Here's how the part is built. I have some questions about the finished solid (model axes, mm). Face numbers are marked on the shaded views. A direction names the side the tool comes from. Round coordinates to 2 decimals unless told otherwise and drop trailing zeros. Order: outer loops, then holes, each group sorted by start corner. A loop starts at its lowest first (then second) coordinate and runs counter-clockwise, first axis right, second up. Notation, with made-up numbers: (85.25, -3) -> (132.25, -3) arc R15 cw to (132.25, 10) -> close; hole circle Ø4 at (7.25, 30). An arc over 180 degrees is marked (long way). One line per item, written item: value.
```python
from build123d import *

# Parameters (mm, degrees)
BOSS_EXTRUDE1_DEPTH = 12.7
SKETCH4_W           = 86.8
SKETCH4_H           = 86.8
SKETCH4_R           = 25.4
BOSS_EXTRUDE3_DEPTH = 340
SKETCH6_W           = 86.8
SKETCH6_H           = 62
CUT_EXTRUDE3_DEPTH  = 12
SKETCH7_W           = 62
SKETCH7_H           = 74.8
CUT_EXTRUDE4_DEPTH  = 12
SKETCH8_W           = 62
SKETCH8_H           = 74.8
CUT_EXTRUDE5_DEPTH  = 12
FILLET2_R           = 35


with BuildPart() as part:
    # Sketch1 → Boss-Extrude1 (new body)
    with BuildSketch(Plane(origin=(0, 0, 0), x_dir=(1, 0, 0), z_dir=(0, 1, 0))):
        Polygon((-367.549574024, 171.211944752), (132.450425976, 171.211944752), (132.450425976, -168.788055248), (-367.549574024, -168.788055248), (-367.549574024, -82.788055248), (7.450425976, -82.788055248), (7.450425976, 85.211944752), (-367.549574024, 85.211944752), align=None)
    extrude(amount=BOSS_EXTRUDE1_DEPTH)

    # Sketch4 → Boss-Extrude3 (add)
    with BuildSketch(Plane.XY.offset(168.788055248)):
        with Locations((50.850425976, 56.1)):
            Rectangle(SKETCH4_W, SKETCH4_H)
        with Locations((50.850425976, 56.1)):
            Circle(SKETCH4_R, mode=Mode.SUBTRACT)
    extrude(amount=-BOSS_EXTRUDE3_DEPTH)

    # Sketch6 → Cut-Extrude3 (cut)
    with BuildSketch(Plane(origin=(0, 99.5, 0), x_dir=(1, 0, 0), z_dir=(0, 1, 0))):
        with Locations((50.850425976, 128.211944752)):
            Rectangle(SKETCH6_W, SKETCH6_H)
    extrude(amount=-CUT_EXTRUDE3_DEPTH, mode=Mode.SUBTRACT)

    # Sketch7 → Cut-Extrude4 (cut)
    with BuildSketch(Plane.ZY.offset(-7.450425976)):
        with Locations((-128.211944752, 50.1)):
            Rectangle(SKETCH7_W, SKETCH7_H)
    extrude(amount=-CUT_EXTRUDE4_DEPTH, mode=Mode.SUBTRACT)

    # Sketch8 → Cut-Extrude5 (cut)
    with BuildSketch(Plane(origin=(94.250425976, 0, 0), x_dir=(0, 0, -1), z_dir=(1, 0, 0))):
        with Locations((128.211944752, 50.1)):
            Rectangle(SKETCH8_W, SKETCH8_H)
    extrude(amount=-CUT_EXTRUDE5_DEPTH, mode=Mode.SUBTRACT)

    # Fillet2
    # the kernel refuses this fillet: 35 mm, written as the material it takes off along each edge
    with BuildSketch(Plane(origin=(82.250425976, 87.5, -97.211944752), x_dir=(-1, 0, 0), z_dir=(0, 0, -1))) as fillet2_piece_1:
        with BuildLine():
            CenterArc((FILLET2_R, -FILLET2_R), FILLET2_R, 90, 90)
            Line((0, -FILLET2_R), (0, 0))
            Line((0, 0), (FILLET2_R, 0))
        make_face()
    extrude(amount=62, mode=Mode.SUBTRACT)
    with BuildSketch(Plane(origin=(19.450425976, 87.5, -159.211944752), x_dir=(0, -1, 0), z_dir=(0, 0, 1))) as fillet2_piece_2:
        with BuildLine():
            CenterArc((FILLET2_R, FILLET2_R), FILLET2_R, 180, 90)
            Line((0, FILLET2_R), (0, 0))
            Line((0, 0), (FILLET2_R, 0))
        make_face()
    extrude(amount=62, mode=Mode.SUBTRACT)


solid = part.part
```
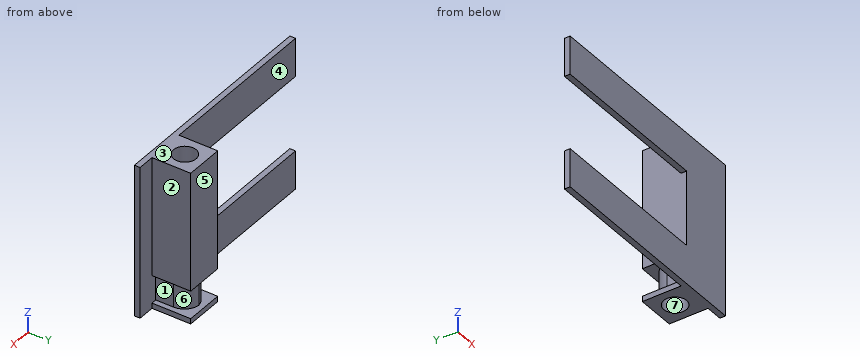
Q1. Which directions (+Z, -Z, +X, -X, +Y, -Y) give clear straight access to the entire face, cutting with the end or side of a thin tool? Please do the marked faces 1, 2, 3 and 4.
Answers:
face 1: +X, +Y
face 2: +Z, -Z, +X, +Y
face 3: +Z, +X, -X, +Y, -Y
face 4: +Z, -Z, -X, +Y
Q2. I want a section at A-A on x = -223.5. Write out the boundary of the cut face in (y, z).
Answers:
outline: (0, -171.21) -> (12.7, -171.21) -> (12.7, -85.21) -> (0, -85.21) -> close; (0, 82.79) -> (12.7, 82.79) -> (12.7, 168.79) -> (0, 168.79) -> close
Q3. I want a section at B-B on y = 41. Write out the boundary of the cut face in (x, z).
Answers:
outline: (7.45, -171.21) -> (30.43, -171.21) -> (30.43, 168.79) -> (7.45, 168.79) -> (7.45, -97.21) -> (19.45, -97.21) -> (19.45, -159.21) -> (7.45, -159.21) -> close; (71.27, -171.21) -> (94.25, -171.21) -> (94.25, -159.21) -> (82.25, -159.21) -> (82.25, -97.21) -> (94.25, -97.21) -> (94.25, 168.79) -> (71.27, 168.79) -> close
Q4. I want a section at C-C on z = -63.5. Write out the boundary of the cut face in (x, y), then the cut area to 3 significant figures.
Answers:
outline: (7.45, 0) -> (132.45, 0) -> (132.45, 12.7) -> (94.25, 12.7) -> (94.25, 99.5) -> (7.45, 99.5) -> close; hole circle Ø50.8 at (50.85, 56.1)
area: 7,090 mm2
Q5. For P1, Ø12, axis at x = 5.5, z = 98.5, coming from the +Y side; P2, Ø5, axis at y = 38, z = -74, coming from the -X side; P3, Ø5, axis at y = 74, z = -16, coming from the +X side; P4, Ø20, axis at y = 34.5, z = -131, coming from the -X side, each with a flat end and sliding along its axis, tell me the tip position at first contact or that it passes through.
Answers:
P1: y = 99.5
P2: x = 7.45
P3: x = 94.25
P4: x = 19.45
Q6. I need wall thicknesses on line 1 along Z through (x, y) = (72.5, 81.5); line 2 along X through (y, z) = (58, 104.5); line 3 along Y through (x, z) = (-191, 83.5). Which ranges of each line are inside material? Lowest first, please.
Answers:
line 1: -171.21 to -159.21, -97.21 to 168.79
line 2: 7.45 to 25.52, 76.18 to 94.25
line 3: 0 to 12.7
Q7. If we mould it in two halves opening along X, with no side actions, what happens to the marked faces 5, 6 and 7? For each: pulls with the +X half, pulls with the -X half, needs draft (parallel to the pull), parting line crosses it, or undercut.
Answers:
face 5: needs draft
face 6: pulls with the +X half
face 7: undercut
